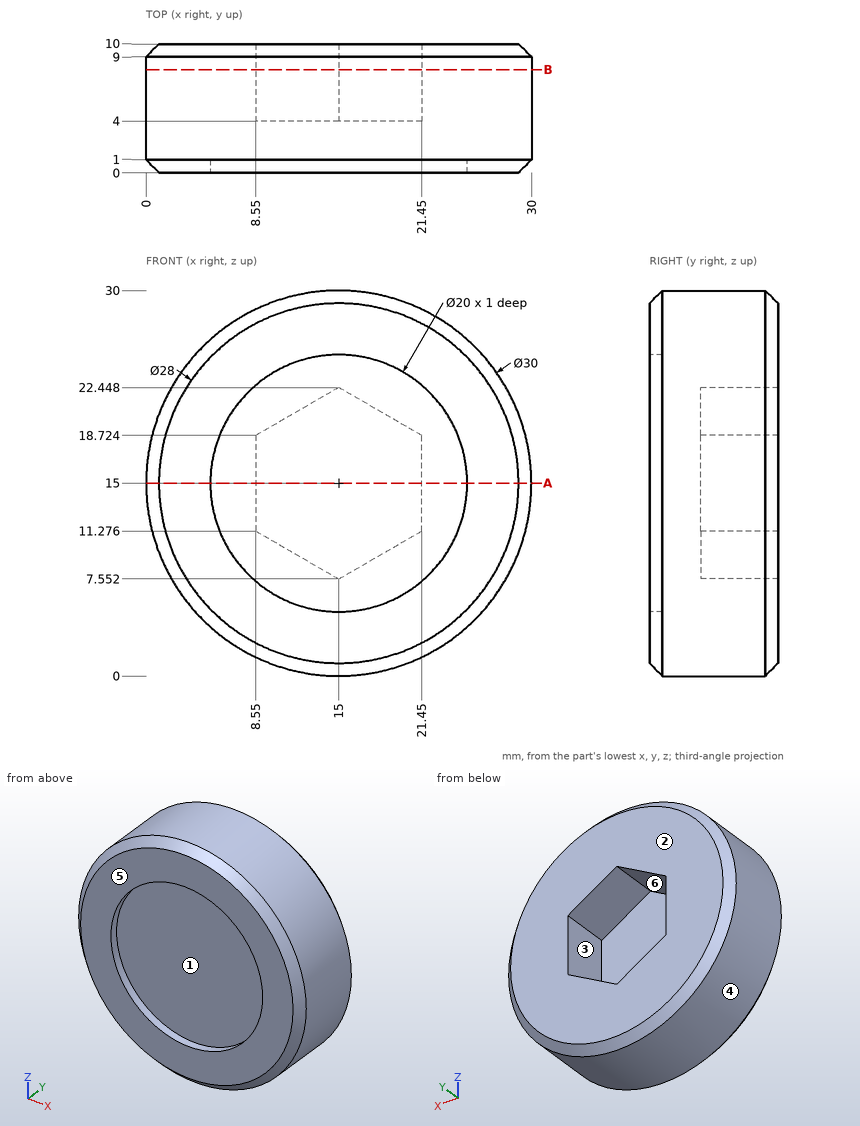
Could you check a few things on this drawing? It's one solid part, dimensions in mm from its lowest x, y, z. A direction names the side the tool comes from. Give positions to 0.01 mm unless a question says otherwise; leave off trailing zeros. Order: outer loops, then holes, each group sorted by start corner. A loop starts at its lowest first (then second) coordinate and runs counter-clockwise, first axis right, second up.
1. For pin 1 (1 mm diameter, centred on x = 19, y = 4, fed in from -Z); pin 2 (1.8 mm diameter, centred on y = 7, z = 16.5, fed in from -X); pin 3 (4 mm diameter, centred on y = 8, z = 23, fed in from -X), each with a flat end and sliding along its axis, tell me the tip position at first contact or that it passes through.
Answers below:
pin 1: stops at z = 0.41
pin 2: stops at x = 0.01
pin 3: stops at x = 1.25
2. I need wall thicknesses on L1, parallel to Z at x = 15, y = 0.3; L2, parallel to X at y = 4.75, z = 14.5; L3, parallel to Z at x = 10, y = 0.75. Which ranges of each line are inside material? Lowest first, please.
Answers below:
L1: z = 0.7 to 5, 25 to 29.3
L2: x = 0.01 to 8.55, 21.45 to 29.99
L3: z = 1.12 to 6.34, 23.66 to 28.88
3. Suppose I cut it at B-B (y = 8). Write out the boundary of the cut face in (x, z).
Answers below:
outline: circle Ø30 at (15, 15); hole (8.55, 11.28) - (15, 7.55) - (21.45, 11.28) - (21.45, 18.72) - (15, 22.45) - (8.55, 18.72) - close
4. Suppose I cut it at A-A (z = 15). Write out the boundary of the cut face in (x, y), plus the area to 3 significant figures.
Answers below:
outline: (0, 1) - (1, 0) - (5, 0) - (5, 1) - (25, 1) - (25, 0) - (29, 0) - (30, 1) - (30, 9) - (29, 10) - (21.45, 10) - (21.45, 4) - (8.55, 4) - (8.55, 10) - (1, 10) - (0, 9) - close
area: 201 mm2
5. Which directions (+Z, -Z, +X, -X, +Y, -Y) give clear straight access to the entire face, cutting with the end or side of a thin tool? Please do the marked faces 1, 2 and 3.
Answers below:
face 1: -Y
face 2: +Z, -Z, +X, -X, +Y
face 3: +Y
6. Thinking about a two-plate mould opening in X: for the marked faces 4, 5 and 6, which applies, +X half, -X half, draft (parallel to the pull), parting line (faces both ways), or undercut?
Answers below:
face 4: parting line
face 5: draft
face 6: undercut
